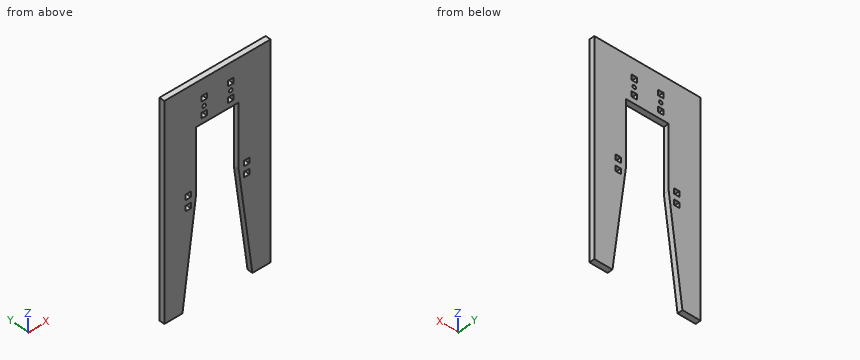
```python
from build123d import *

# Parameters (mm, degrees)
BOTTOM_PLATE_R      = 2.159
BOTTOM_PLATE_R_2    = 2.794
BOTTOM_PLATE_W      = 25.4
BOTTOM_PLATE_H      = 101.6
BOTTOM_PLATE_W_2    = 6.35
BOTTOM_PLATE_H_2    = 6.35
BOSS_EXTRUDE1_DEPTH = 6.35
SKETCH1_W           = 508
SKETCH1_H           = 508
SKETCH1_W_2         = 127
SKETCH1_H_2         = 254
CUT_EXTRUDE2_DEPTH  = 25.4


with BuildPart() as part:
    # Bottom Plate → Boss-Extrude1 (new body)
    # profile 1 of 3: a face of its own
    with BuildSketch(Plane(origin=(0, 0, 0), x_dir=(1, 0, 0), z_dir=(0, 1, 0))):
        with BuildLine():
            Line((25.4, 0), (50.8, 196.747553987))
            ThreePointArc((50.8, 196.747553987), (0, -203.2), (-50.8, 196.747553987))
            Line((-50.8, 196.747553987), (-25.4, 0))
            Line((-25.4, 0), (-25.4, -76.2))
            Line((-25.4, -76.2), (25.4, -76.2))
            Line((25.4, -76.2), (25.4, 0))
        make_face()
        with Locations((155.026770144, 72.009)):
            Circle(BOTTOM_PLATE_R, mode=Mode.SUBTRACT)
        with Locations((155.026770144, -72.009)):
            Circle(BOTTOM_PLATE_R, mode=Mode.SUBTRACT)
        with Locations((57.243949466, 172.269543754)):
            Circle(BOTTOM_PLATE_R, mode=Mode.SUBTRACT)
        with Locations(Location((-15.875, -95.25, 0), (0, 0, 270))):
            Circle(BOTTOM_PLATE_R, mode=Mode.SUBTRACT)
        with Locations((27.813, -152.4)):
            Circle(BOTTOM_PLATE_R_2, mode=Mode.SUBTRACT)
        with Locations((-27.813, -152.4)):
            Circle(BOTTOM_PLATE_R_2, mode=Mode.SUBTRACT)
        with Locations(Location((15.875, -95.25, 0), (0, 0, 90))):
            Circle(BOTTOM_PLATE_R, mode=Mode.SUBTRACT)
        with Locations((-155.026770144, -72.009)):
            Circle(BOTTOM_PLATE_R, mode=Mode.SUBTRACT)
        with Locations((-155.026770144, 72.009)):
            Circle(BOTTOM_PLATE_R, mode=Mode.SUBTRACT)
        with Locations((-57.243949466, 172.269543754)):
            Circle(BOTTOM_PLATE_R, mode=Mode.SUBTRACT)
        with Locations((170.901770144, 0)):
            Rectangle(BOTTOM_PLATE_W, BOTTOM_PLATE_H, mode=Mode.SUBTRACT)
        with Locations((-34.925, 9.525)):
            Rectangle(BOTTOM_PLATE_W_2, BOTTOM_PLATE_H_2, mode=Mode.SUBTRACT)
        with Locations((34.925, -3.175)):
            Rectangle(BOTTOM_PLATE_W_2, BOTTOM_PLATE_H_2, mode=Mode.SUBTRACT)
        with Locations((34.925, 9.525)):
            Rectangle(BOTTOM_PLATE_W_2, BOTTOM_PLATE_H_2, mode=Mode.SUBTRACT)
        with Locations((155.026770144, -60.325)):
            Rectangle(BOTTOM_PLATE_W_2, BOTTOM_PLATE_H_2, mode=Mode.SUBTRACT)
        with Locations((155.026770144, 60.325)):
            Rectangle(BOTTOM_PLATE_W_2, BOTTOM_PLATE_H_2, mode=Mode.SUBTRACT)
        with Locations((-34.925, -3.175)):
            Rectangle(BOTTOM_PLATE_W_2, BOTTOM_PLATE_H_2, mode=Mode.SUBTRACT)
        with Locations((-15.875, -85.725)):
            Rectangle(BOTTOM_PLATE_W_2, BOTTOM_PLATE_H_2, mode=Mode.SUBTRACT)
        with Locations((-15.875, -104.775)):
            Rectangle(BOTTOM_PLATE_W_2, BOTTOM_PLATE_H_2, mode=Mode.SUBTRACT)
        with Locations((15.875, -104.775)):
            Rectangle(BOTTOM_PLATE_W_2, BOTTOM_PLATE_H_2, mode=Mode.SUBTRACT)
        with Locations((15.875, -85.725)):
            Rectangle(BOTTOM_PLATE_W_2, BOTTOM_PLATE_H_2, mode=Mode.SUBTRACT)
        with Locations((-170.901770144, 0)):
            Rectangle(BOTTOM_PLATE_W, BOTTOM_PLATE_H, mode=Mode.SUBTRACT)
        with Locations((-155.026770144, -60.325)):
            Rectangle(BOTTOM_PLATE_W_2, BOTTOM_PLATE_H_2, mode=Mode.SUBTRACT)
        with Locations((-155.026770144, 60.325)):
            Rectangle(BOTTOM_PLATE_W_2, BOTTOM_PLATE_H_2, mode=Mode.SUBTRACT)
    # profile 2 of 3: a face of its own
    with BuildSketch(Plane(origin=(0, 0, 0), x_dir=(1, 0, 0), z_dir=(0, 1, 0))):
        Polygon((55.672367921, 184.893668177), (61.970103658, 184.08063399), (62.783137846, 190.378369726), (56.485402109, 191.191403914), align=None)
    # profile 3 of 3: a face of its own
    with BuildSketch(Plane(origin=(0, 0, 0), x_dir=(1, 0, 0), z_dir=(0, 1, 0))):
        Polygon((-61.970103658, 184.08063399), (-62.783137846, 190.378369726), (-56.485402109, 191.191403914), (-55.672367921, 184.893668177), align=None)
    extrude(amount=-BOSS_EXTRUDE1_DEPTH)

    # Sketch1 → Cut-Extrude2 (cut)
    with BuildSketch(Plane(origin=(0, 0, 0), x_dir=(1, 0, 0), z_dir=(0, 1, 0))):
        Rectangle(SKETCH1_W, SKETCH1_H)
        Rectangle(SKETCH1_W_2, SKETCH1_H_2, mode=Mode.SUBTRACT)
    extrude(amount=-CUT_EXTRUDE2_DEPTH, mode=Mode.SUBTRACT)


solid = part.part
```
Here's how the part is built. I have some questions about the finished solid (model axes, mm). Give positions to 0.01 mm unless a question says otherwise; leave off trailing zeros. Loops run counter-clockwise (first coordinate to the right, second up) from the corner with the lowest first, then second, coordinate; pieces in that order, holes last. Notation, with made-up numbers: M 54.5,56.25 L 58.5,56.25 A16 ccw 58.5,82.25 Z; hole C -22.75,83.25 d2. An arc over 180 degrees is marked long. Put each result on its own line as item: value. Start each with the question number.
(1) I want a section at A-A on z = -34.5. Please give me the cut outline in (x, y), then the cut area to 3 significant figures.
(2) Will these pins go through, and if not, where does the flat tip stop? pin 1 Ø1.5 at (x, z) = (-23, 52.5) entering from -Y; pin 2 Ø1.9 at (x, y) = (17, -2) entering from -Z.
(3) I need wall thicknesses on line 1 along X through (y, z) = (-3.5, 95.25); line 2 along X through (y, z) = (-2.75, 12.5); line 3 along Z through (x, y) = (-1, -1). Which ranges of each line are inside material? Lowest first, please. Write a range as [from, to].
(4) I want a section at C-C on y = -3. State how many separate pieces and enclosed holes the cut face has, then the cut area to 3 significant figures.
(5) I want a section at B-B on x = -6. Please give me the cut outline in (y, z), then the cut area to 3 significant figures.
Answer block:
1. outline: M -63.5,-6.35 L -29.85,-6.35 L -29.85,0 L -63.5,0 Z; M 29.85,-6.35 L 63.5,-6.35 L 63.5,0 L 29.85,0 Z
1. area: 427 mm^2
2. pin 1: through
2. pin 2: z = 76.2
3. line 1: [-63.5, -18.03], [-13.72, 13.72], [18.03, 63.5]
3. line 2: [-63.5, -25.4], [25.4, 63.5]
3. line 3: [76.2, 127]
4. separate pieces: 1
4. enclosed holes: 10
4. area: 19,500 mm^2
5. outline: M -6.35,76.2 L 0,76.2 L 0,127 L -6.35,127 Z
5. area: 323 mm^2
